Could you check a few things on this model? Use its own coordinates, in mm. A direction names the side the tool comes from. Give positions to 0.01 mm unless a question says otherwise; leave off trailing zeros. Loops run counter-clockwise (first coordinate to the right, second up) from the corner with the lowest first, then second, coordinate; pieces in that order, holes last. Notation, with made-up numbers: M 33,86 L 64,86 A22 cw 64,117 Z; hole C 79.25,-5.75 d10. An arc over 180 degrees is marked long. Use CSV: the item, a comma, the result in double quotes.
```python
from build123d import *

# Parameters (mm, degrees)
SKETCH1_W                = 25.4
SKETCH1_H                = 25.4
SKETCH1_W_2              = 19.05
SKETCH1_H_2              = 19.05
BOSS_EXTRUDE1_DEPTH      = 228.6
BOSS_EXTRUDE1_DEPTH_BACK = 38.1
CUT_EXTRUDE2_REACH       = 27.4
SKETCH3_W                = 10.16
SKETCH3_H                = 76.2
SKETCH4_R                = 3.175
SKETCH4_R_2              = 2.38125
SKETCH4_R_3              = 4.7625
CUT_EXTRUDE3_DEPTH       = 26.4


with BuildPart() as part:
    # Sketch1 → Boss-Extrude1 (new body, two sides)
    with BuildSketch(Plane(origin=(0, 0, 0), x_dir=(1, 0, 0), z_dir=(0, 1, 0))) as boss_extrude1_sk:
        Rectangle(SKETCH1_W, SKETCH1_H)
        Rectangle(SKETCH1_W_2, SKETCH1_H_2, mode=Mode.SUBTRACT)
    extrude(amount=BOSS_EXTRUDE1_DEPTH)
    extrude(boss_extrude1_sk.sketch, amount=-BOSS_EXTRUDE1_DEPTH_BACK)

    # Sketch3 → Cut-Extrude2 (cut, up to next)
    with BuildSketch(Plane(origin=(0, 0, -12.7), x_dir=(-1, 0, 0), z_dir=(0, 0, -1)), mode=Mode.PRIVATE) as cut_extrude2_sk1:
        with Locations((0, 82.55)):
            Rectangle(SKETCH3_W, SKETCH3_H)
    cut_extrude2_tool1 = extrude(cut_extrude2_sk1.sketch, amount=-CUT_EXTRUDE2_REACH, mode=Mode.PRIVATE) & part.part
    add(cut_extrude2_tool1.solids().sort_by_distance((0, 82.55, -12.7))[0], mode=Mode.SUBTRACT)

    # Sketch4 → Cut-Extrude3 (cut, through all)
    with BuildSketch(Plane(origin=(12.7, 0, 0), x_dir=(0, 0, -1), z_dir=(1, 0, 0))):
        with Locations((3.175, -28.575)):
            Circle(SKETCH4_R)
        with Locations((3.175, -12.7)):
            Circle(SKETCH4_R)
        with Locations((0, 63.246)):
            Circle(SKETCH4_R_2)
        with Locations((0, 72.898)):
            Circle(SKETCH4_R_2)
        with Locations((0, 82.55)):
            Circle(SKETCH4_R_2)
        with Locations((0, 101.854)):
            Circle(SKETCH4_R_2)
        with Locations((0, 111.506)):
            Circle(SKETCH4_R_2)
        with Locations((0, 12.7)):
            Circle(SKETCH4_R_3)
        with Locations((0, 53.594)):
            Circle(SKETCH4_R_2)
        with Locations((0, 92.202)):
            Circle(SKETCH4_R_2)
    extrude(amount=-CUT_EXTRUDE3_DEPTH, mode=Mode.SUBTRACT)


solid = part.part
```
1. Which directions (+Z, -Z, +X, -X, +Y, -Y) give clear straight access to the entire face, cutting with the end or side of a thin tool? Please do faces 1 (the face through (11.135, 70.573, 0.516)), 2 (the face through (9.525, 97, 0)).
Outcome:
face 1,"+X, -X"
face 2,"+Y, -Y"
2. I want a section at A-A, the plane y = 12.7. List the corners of the cut face in (x, z) for me (1 decimal).
Outcome:
outline,"M -12.7,-12.7 L 12.7,-12.7 L 12.7,-4.8 L 9.5,-4.8 L 9.5,-9.5 L -9.5,-9.5 L -9.5,-4.8 L -12.7,-4.8 Z; M -12.7,4.8 L -9.5,4.8 L -9.5,9.5 L 9.5,9.5 L 9.5,4.8 L 12.7,4.8 L 12.7,12.7 L -12.7,12.7 Z"
3. If we mould it in two halves opening along X, with no side actions, what happens to faces 3 (the face through (0, 97, 9.525)), 4 (the face through (-11.09, 89.88, 0.52))? For each: +X half, -X half, draft (parallel to the pull), parting line (faces both ways), or undercut.
Outcome:
face 3,"undercut"
face 4,"draft"
4. Please list where these lines run through material, in increasing order: line 1 (Z direction, x = -9.25, y = 166.5) (3 decimals); line 2 (X direction, y = 51, z = -11).
Outcome:
line 1,"-12.7 to -9.525, 9.525 to 12.7"
line 2,"-12.7 to -5.08, 5.08 to 12.7"
5. I want a section at C-C, the plane y = 152.5. List the corners of the cut face in (x, z) for me (3 decimals), then the cut area to 3 significant figures.
Outcome:
outline,"M -12.7,-12.7 L 12.7,-12.7 L 12.7,12.7 L -12.7,12.7 Z; hole M -9.525,-9.525 L 9.525,-9.525 L 9.525,9.525 L -9.525,9.525 Z"
area,"282 mm2"
6. I want a section at B-B, the plane y = 82.55. List the corners of the cut face in (x, z) for me (3 decimals), then the cut area to 3 significant figures.
Outcome:
outline,"M -12.7,-12.7 L -5.08,-12.7 L -5.08,-9.525 L -9.525,-9.525 L -9.525,-2.381 L -12.7,-2.381 Z; M -12.7,2.381 L -9.525,2.381 L -9.525,9.525 L 9.525,9.525 L 9.525,2.381 L 12.7,2.381 L 12.7,12.7 L -12.7,12.7 Z; M 5.08,-12.7 L 12.7,-12.7 L 12.7,-2.381 L 9.525,-2.381 L 9.525,-9.525 L 5.08,-9.525 Z"
area,"220 mm2"
7. I'm going to push a flat-ended pin straight in: pin 1 Ø6 at (x, z) = (4, 4) entering from -Y. Where does the tip first touch, or does it pass through?
Outcome:
pin 1,"through"
